Model file for the job. Use its own axes, mm. Face numbers are marked on the shaded views. Give positions to 0.01 mm unless a question says otherwise; leave off trailing zeros. Order: outer loops, then holes, each group sorted by start corner. A loop starts at its lowest first (then second) coordinate and runs counter-clockwise, first axis right, second up. Notation, with made-up numbers: M 43,2.5 L 95,2.5 A24 cw 95,26.5 Z; hole C 8,67 d4. An arc over 180 degrees is marked long. Return JSON: item names as keys, results as strings. Group by question number.
1. Slice it at C-C on y = 83.75. List the corners of the cut face in (x, z).
2. Two-plate mould, pull along Y, no slides. Class the marked faces 1, 2 and 3: released by +Y, released by -Y, zero draft, split by the parting line, or undercut.
3. Slice it at B-B on z = 9.25. List the corners of the cut face in (x, y).
4. Slice it at A-A on x = -31.25. List the corners of the cut face in (y, z), then the cut area to 3 significant figures.
5. Wall check: probe 1 along X at (y, z) = (91, 9.25); probe 2 along X at (y, z) = (92.05, -9.25); probe 3 along X at (y, z) = (72.25, 5). Give the ranges that are in metal, low to high. Write a range as [from, to].
6. Slice it at D-D on z = 3. List the corners of the cut face in (x, y).
7. Pin check, flat tips, straight feed: pin 1 (1.6 mm diameter, centred on x = 31.5, y = 91.5, fed in from -Z); pin 2 (1 mm diameter, centred on y = 79, z = -3.5, fed in from +X); pin 3 (5 mm diameter, centred on y = 84.5, z = 4, fed in from -X). Stop position of each tip, or through.
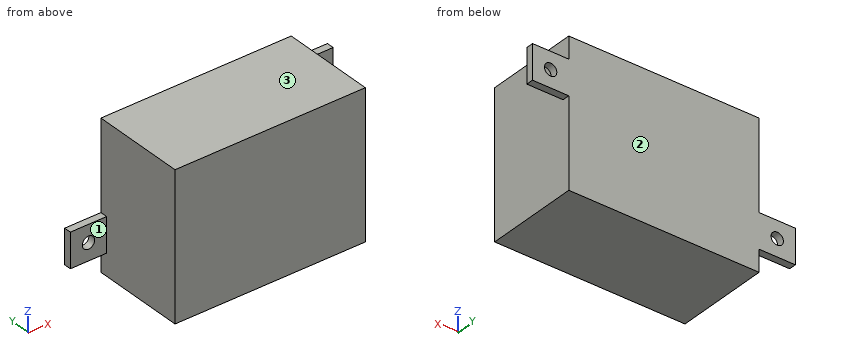
from build123d import *

# Parameters (mm, degrees)
CASE_START    = 66.57
CASE_SKETCH_W = 52.5
CASE_SKETCH_H = 40
CASE_2_DEPTH  = 26
EARS_START    = 90.57
EARS_SKETCH_W = 10
EARS_SKETCH_H = 9.5
EARS_SKETCH_R = 1.7
EARS_DEPTH    = 2


with BuildPart() as part:
    # Case Sketch → Case 2 (new body)
    with BuildSketch(Plane(origin=(0, 0, 0), x_dir=(1, 0, 0), z_dir=(0, 1, 0)).offset(CASE_START)):
        Rectangle(CASE_SKETCH_W, CASE_SKETCH_H)
    extrude(amount=CASE_2_DEPTH)

    # Ears Sketch → Ears (add)
    # profile 1 of 2: a face of its own
    with BuildSketch(Plane(origin=(0, 0, 0), x_dir=(1, 0, 0), z_dir=(0, 1, 0)).offset(EARS_START)):
        with Locations((31.25, -9.25)):
            Rectangle(EARS_SKETCH_W, EARS_SKETCH_H)
        with Locations(Location((31.25, -9.25, 0), (0, 0, 270))):
            Circle(EARS_SKETCH_R, mode=Mode.SUBTRACT)
    # profile 2 of 2: a face of its own
    with BuildSketch(Plane(origin=(0, 0, 0), x_dir=(1, 0, 0), z_dir=(0, 1, 0)).offset(EARS_START)):
        with Locations((-31.25, 9.25)):
            Rectangle(EARS_SKETCH_W, EARS_SKETCH_H)
        with Locations(Location((-31.25, 9.25, 0), (0, 0, 270))):
            Circle(EARS_SKETCH_R, mode=Mode.SUBTRACT)
    extrude(amount=EARS_DEPTH)


solid = part.part
Result:
{
 "1": {"outline": "M -26.25,-20 L 26.25,-20 L 26.25,20 L -26.25,20 Z"},
 "2": {"face 1": "released by -Y", "face 2": "released by +Y", "face 3": "zero draft"},
 "3": {"outline": "M -26.25,66.57 L 26.25,66.57 L 26.25,90.57 L 29.55,90.57 L 29.55,92.57 L -26.25,92.57 Z; M 32.95,90.57 L 36.25,90.57 L 36.25,92.57 L 32.95,92.57 Z"},
 "4": {"outline": "M 90.57,-14 L 92.57,-14 L 92.57,-10.95 L 90.57,-10.95 Z; M 90.57,-7.55 L 92.57,-7.55 L 92.57,-4.5 L 90.57,-4.5 Z", "area": "12.2 mm2"},
 "5": {"probe 1": "x = [-26.25, 29.55], [32.95, 36.25]", "probe 2": "x = [-36.25, -32.95], [-29.55, 26.25]", "probe 3": "x = [-26.25, 26.25]"},
 "6": {"outline": "M -26.25,66.57 L 26.25,66.57 L 26.25,92.57 L -26.25,92.57 Z"},
 "7": {"pin 1": "stops at z = 4.5", "pin 2": "stops at x = 26.25", "pin 3": "stops at x = -26.25"}
}
